Geometry check sheet. Reference: drawing and pictorial views, mm from the part's lowest x, y, z. A direction names the side the tool comes from. Give positions to 0.01 mm unless a question says otherwise; leave off trailing zeros. Write each loop counter-clockwise with the first axis right and the second up, starting at its lowest first coordinate (ties: lowest second). Pieces come first, ordered by that corner, then holes. Notation, with made-up numbers: (54.5, 3) - (67.5, 3) arc R25 ccw to (67.5, 26) - close; hole circle Ø9 at (88, -16.75). An arc over 180 degrees is marked (long way). Write item = value, one per line. Start each with the question number.
(1) Section check A-A, the plane y = 7.5. Enter the section's corners in (x, z), plus the area to 3 significant figures.
(2) Access from +Z, -Z, +X, -X, +Y, -Y to the whole of each face (thin tool, end or side, straight path). Record for the marked faces 1, 2 and 3.
(3) Section check D-D, the plane z = 32.5. Enter the section's corners in (x, y).
(4) Section check C-C, the plane z = 7. Enter the section's corners in (x, y), plus the area to 3 significant figures.
(5) Thickness scan on L1, parallel to Y at x = 7.5, z = 20.5; L2, parallel to Z at x = 4, y = 12.5; L3, parallel to Y at x = 12, z = 39.5. Record the ranges inside material, lowest first.
(6) Depth check by flat-ended pin: pin 1 Ø4 at (y, z) = (12, 10.5) entering from +X; pin 2 Ø6 at (y, z) = (7, 22.5) entering from +X; pin 3 Ø2 at (x, y) = (10, 11.5) entering from +Z. Enter the tip coordinate at first touch or a pass-through.
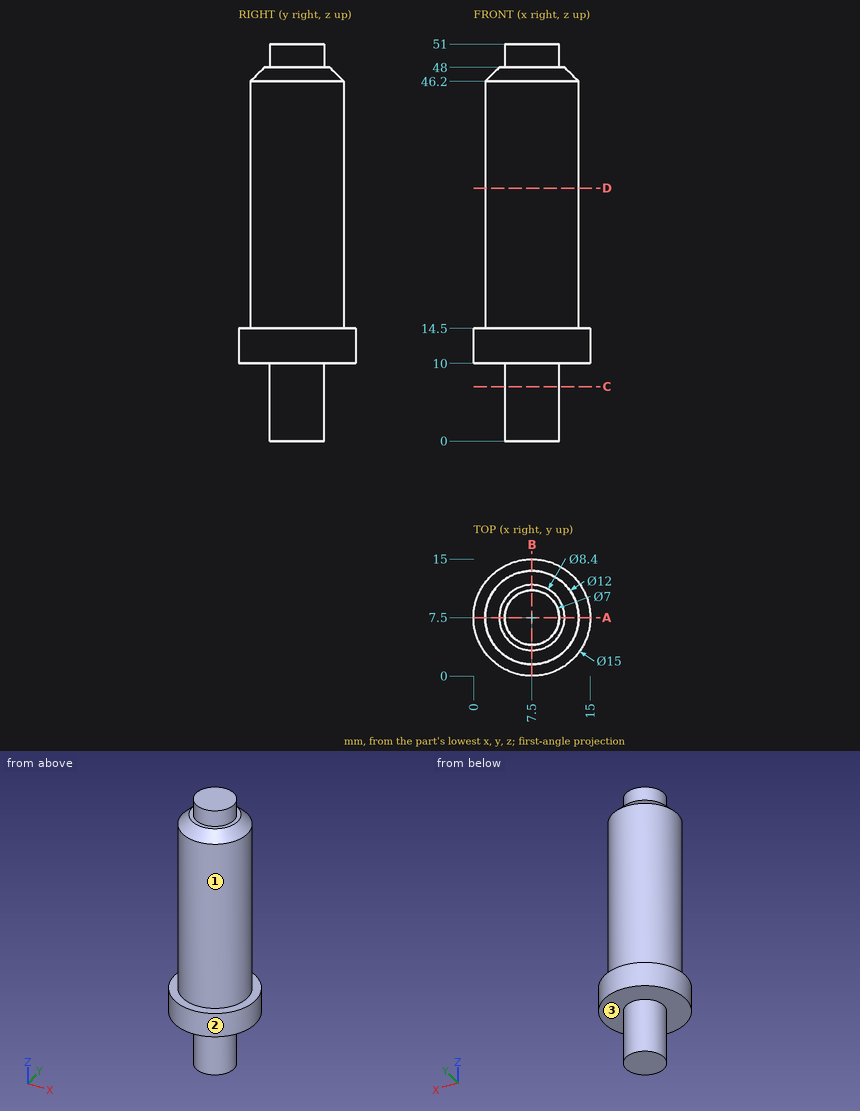
Model answer:
q1.outline = (0, 10) - (4, 10) - (4, 0) - (11, 0) - (11, 10) - (15, 10) - (15, 14.5) - (13.5, 14.5) - (13.5, 46.2) - (11.7, 48) - (11, 48) - (11, 51) - (4, 51) - (4, 48) - (3.3, 48) - (1.5, 46.2) - (1.5, 14.5) - (0, 14.5) - close
q1.area = 557 mm²
q2.face_1 = +Z
q2.face_2 = +Z, -Z
q2.face_3 = -Z
q3.outline = circle Ø12 at (7.5, 7.5)
q4.outline = circle Ø7 at (7.5, 7.5)
q4.area = 38.5 mm²
q5.L1 = 1.5 to 13.5
q5.L2 = 10 to 14.5
q5.L3 = 3.53 to 11.47
q6.pin_1 = 14.57
q6.pin_2 = 13.5
q6.pin_3 = 48
